```python
from build123d import *

# Parameters (mm, degrees)
SKETCH1_R           = 180
BOSS_EXTRUDE1_DEPTH = 60
FILLET1_R           = 20
SKETCH2_R           = 100
BOSS_EXTRUDE3_DEPTH = 10
SKETCH3_R           = 90
BOSS_EXTRUDE4_DEPTH = 270
SKETCH4_R           = 180
BOSS_EXTRUDE5_DEPTH = 60
FILLET2_R           = 30
BOSS_EXTRUDE6_START = 10
SKETCH6_R           = 100
BOSS_EXTRUDE6_DEPTH = 10
FILLET3_R           = 5
SKETCH9_W           = 20.845427705
SKETCH9_H           = 31.268141557
BOSS_EXTRUDE7_DEPTH = 10
SKETCH10_R          = 10
CUT_EXTRUDE2_DEPTH  = 10
CUT_EXTRUDE3_START  = 10
SKETCH12_R          = 10
CUT_EXTRUDE3_DEPTH  = 10
SKETCH13_RX         = 11.260558061
SKETCH13_RY         = 5.777483036
CUT_EXTRUDE4_DEPTH  = 30
SKETCH14_W          = 10.93815799
SKETCH14_H          = 4.07197177
SKETCH14_W_2        = 12.726253657
CUT_EXTRUDE5_DEPTH  = 30
FILLET4_START       = -31
FILLET4_DEPTH       = 62
FILLET4_START_2     = -9.089801569
FILLET4_2_DEPTH     = 40.089801569
CUT_EXTRUDE6_DEPTH  = 10
CUT_EXTRUDE7_DEPTH  = 10


with BuildPart() as part:
    # Sketch1 → Boss-Extrude1 (new body)
    with BuildSketch(Plane(origin=(0, 0, 0), x_dir=(1, 0, 0), z_dir=(0, 1, 0))):
        with Locations(Location((0, 0, 0), (0, 0, 90))):
            Circle(SKETCH1_R)
    extrude(amount=BOSS_EXTRUDE1_DEPTH)

    # Fillet1
    fillet1_edges = [part.edges().sort_by_distance(p)[0] for p in [
        (0, 0, 180),
    ]]
    fillet(fillet1_edges, radius=FILLET1_R)

    # Sketch2 → Boss-Extrude3 (add)
    with BuildSketch(Plane(origin=(0, 60, 0), x_dir=(1, 0, 0), z_dir=(0, 1, 0))):
        with Locations(Location((0, 0, 0), (0, 0, 270))):
            Circle(SKETCH2_R)
    extrude(amount=BOSS_EXTRUDE3_DEPTH)

    # Sketch3 → Boss-Extrude4 (add)
    with BuildSketch(Plane(origin=(0, 70, 0), x_dir=(1, 0, 0), z_dir=(0, 1, 0))):
        with Locations(Location((0, 0, 0), (0, 0, 270))):
            Circle(SKETCH3_R)
    extrude(amount=BOSS_EXTRUDE4_DEPTH)

    # Sketch4 → Boss-Extrude5 (add)
    with BuildSketch(Plane(origin=(0, 340, 0), x_dir=(1, 0, 0), z_dir=(0, 1, 0))):
        with Locations(Location((0, 0, 0), (0, 0, 90))):
            Circle(SKETCH4_R)
    extrude(amount=BOSS_EXTRUDE5_DEPTH)

    # Fillet2
    fillet2_edges = [part.edges().sort_by_distance(p)[0] for p in [
        (0, 400, 180),
    ]]
    fillet(fillet2_edges, radius=FILLET2_R)

    # Sketch6 → Boss-Extrude6 (add)
    with BuildSketch(Plane.XZ.offset(-340).offset(BOSS_EXTRUDE6_START)):
        with Locations(Location((0, 0, 0), (0, 0, 90))):
            Circle(SKETCH6_R)
    extrude(amount=-BOSS_EXTRUDE6_DEPTH)

    # Fillet3
    fillet3_edges = [part.edges().sort_by_distance(p)[0] for p in [
        (0, 330, -100),
        (0, 70, -100),
    ]]
    fillet(fillet3_edges, radius=FILLET3_R)

    # Sketch9 → Boss-Extrude7 (add)
    with BuildSketch(Plane(origin=(0, 60, 0), x_dir=(1, 0, 0), z_dir=(0, 1, 0))):
        with Locations((-19.512515422, -149.90314923)):
            Rectangle(SKETCH9_W, SKETCH9_H)
        with Locations((19.656209668, -149.671177345)):
            Rectangle(SKETCH9_W, SKETCH9_H)
    extrude(amount=BOSS_EXTRUDE7_DEPTH)

    # Sketch10 → Cut-Extrude2 (cut)
    with BuildSketch(Plane.XY.offset(180)):
        with Locations((0, 355)):
            Circle(SKETCH10_R)
    extrude(amount=-CUT_EXTRUDE2_DEPTH, mode=Mode.SUBTRACT)

    # Sketch12 → Cut-Extrude3 (cut)
    with BuildSketch(Plane.XY.offset(-180).offset(CUT_EXTRUDE3_START)):
        with Locations((0, 355)):
            Circle(SKETCH12_R)
    extrude(amount=-CUT_EXTRUDE3_DEPTH, mode=Mode.SUBTRACT)

    # Sketch13 → Cut-Extrude4 (cut)
    with BuildSketch(Plane.ZY.offset(29.935229274)):
        with Locations((149.903149231, 70)):
            Ellipse(SKETCH13_RX, SKETCH13_RY)
    extrude(amount=-CUT_EXTRUDE4_DEPTH, mode=Mode.SUBTRACT)

    # Sketch14 → Cut-Extrude5 (cut)
    with BuildSketch(Plane(origin=(30.07892352, 0, 0), x_dir=(0, 0, -1), z_dir=(1, 0, 0))):
        with Locations((-159.836169129, 67.964014115)):
            Rectangle(SKETCH14_W, SKETCH14_H)
        with Locations((-140.400233395, 67.964014115)):
            Rectangle(SKETCH14_W_2, SKETCH14_H)
    extrude(amount=-CUT_EXTRUDE5_DEPTH, mode=Mode.SUBTRACT)

    # Fillet4: read off the stored shape, not the designer's step
    # Fillet4 outline → Fillet4 (cut)
    with BuildSketch(Plane.YZ.offset(FILLET4_START)):
        with BuildLine():
            Line((70, 165.537220009), (68, 165.537220009))
            ThreePointArc((68, 165.537220009), (69.414213562, 164.951433572), (70, 163.537220009))
            Line((70, 163.537220009), (70, 165.537220009))
        make_face()
        with BuildLine():
            Line((70, 161.163707292), (70, 162.751420247))
            ThreePointArc((70, 162.751420247), (69.666591866, 161.645765891), (68.777528446, 160.908745692))
            add(Edge.make_bspline(
                [(68.777528446, 160.908745692), (69.381765186, 161.163707292), (70, 161.163707292)],
                knots=[6.055563227, 6.055563227, 6.055563227, 6.283185307, 6.283185307, 6.283185307], degree=2, weights=[0.927415097, 0.957557219, 1]))
        make_face()
        with BuildLine():
            Line((70, 154.367090134), (68, 154.367090134))
            ThreePointArc((68, 154.367090134), (69.414213562, 153.781303696), (70, 152.367090134))
            Line((70, 152.367090134), (70, 154.367090134))
        make_face()
        with BuildLine():
            add(Edge.make_bspline(
                [(70, 138.642591169), (69.381765186, 138.642591169), (68.777528446, 138.897552769)],
                knots=[3.141592654, 3.141592654, 3.141592654, 3.369214734, 3.369214734, 3.369214734], degree=2, weights=[1, 0.957557219, 0.927415097]))
            ThreePointArc((68.777528446, 138.897552769), (69.666591866, 138.16053257), (70, 137.054878214))
            Line((70, 137.054878214), (70, 138.642591169))
        make_face()
        with BuildLine():
            ThreePointArc((70, 148.763360224), (69.414213562, 147.349146661), (68, 146.763360224))
            Line((68, 146.763360224), (70, 146.763360224))
            Line((70, 146.763360224), (70, 148.763360224))
        make_face()
        with BuildLine():
            Line((65.92802823, 134.269078452), (64.862948862, 134.269078452))
            ThreePointArc((64.862948862, 134.269078452), (64.409662828, 134.095965635), (63.92802823, 134.037106567))
            Line((63.92802823, 134.037106567), (65.92802823, 134.037106567))
            Line((65.92802823, 134.037106567), (65.92802823, 134.269078452))
        make_face()
        with BuildLine():
            ThreePointArc((70, 136.269078452), (69.414213562, 134.85486489), (68, 134.269078452))
            Line((68, 134.269078452), (70, 134.269078452))
            Line((70, 134.269078452), (70, 136.269078452))
        make_face()
    extrude(amount=FILLET4_DEPTH, mode=Mode.SUBTRACT)

    # Fillet4 2 outline → Fillet4 2 (cut)
    with BuildSketch(Plane.YZ.offset(FILLET4_START_2)):
        with BuildLine():
            ThreePointArc((63.92802823, 165.305248124), (65.342241792, 164.719461686), (65.92802823, 163.305248124))
            Line((65.92802823, 163.305248124), (65.92802823, 165.305248124))
            Line((65.92802823, 165.305248124), (63.92802823, 165.305248124))
        make_face()
        with BuildLine():
            Line((65.92802823, 134.269078452), (65.92802823, 136.037106567))
            ThreePointArc((65.92802823, 136.037106567), (65.641189236, 135.005079741), (64.862948862, 134.269078452))
            Line((64.862948862, 134.269078452), (65.92802823, 134.269078452))
        make_face()
    extrude(amount=FILLET4_2_DEPTH, mode=Mode.SUBTRACT)

    # Sketch22 → Cut-Extrude6 (cut)
    with BuildSketch(Plane(origin=(0, 60, 0), x_dir=(1, 0, 0), z_dir=(0, 1, 0))):
        Polygon((127.423760752, -18.872499432), (107.1351894, -64.521784974), (113.629623838, -67.40820028), (133.91819519, -21.758914738), align=None)
        Polygon((137.220873331, -23.883738258), (116.932301979, -69.5330238), (123.677729052, -72.530991388), (143.966300404, -26.881705846), align=None)
        Polygon((148.265392154, -28.776757418), (127.858476847, -74.692316859), (134.98259987, -77.858593758), (155.389515177, -31.943034317), align=None)
    extrude(amount=-CUT_EXTRUDE6_DEPTH, mode=Mode.SUBTRACT)

    # Sketch24 → Cut-Extrude7 (cut)
    with BuildSketch(Plane(origin=(0, 60, 0), x_dir=(1, 0, 0), z_dir=(0, 1, 0))):
        Polygon((111.713779985, 58.505093082), (105.578926162, 52.370239259), (74.729375507, 83.219789913), (80.86422933, 89.354643737), align=None)
        Polygon((115.569973817, 62.361286914), (84.720423162, 93.210837569), (90.154150834, 98.644565241), (121.003701489, 67.795014586), align=None)
        Polygon((93.930128704, 100.831618279), (123.985216943, 70.77653004), (128.873539941, 75.664853038), (98.818451702, 105.719941277), align=None)
    extrude(amount=-CUT_EXTRUDE7_DEPTH, mode=Mode.SUBTRACT)


solid = part.part
```
Check sheet for the modelled part. Datum: model origin and axes. Units: mm. A direction names the side the tool comes from. Coordinates: 2 decimals unless noted, no trailing zeros. Order: outer loops, then holes, each group sorted by start corner. A loop starts at its lowest first (then second) coordinate and runs counter-clockwise, first axis right, second up. Notation, with made-up numbers: M 17,69.5 L 58,69.5 A29 cw 58,93.5 Z; hole C -36.5,27 d2. An arc over 180 degrees is marked long. Write each question's results on one line, items separated by ' | '. Start each with the question number.
1. Cross-section at B-B on y = 198. Record the cut outline in (x, z), and give its area (3 significant figures).
2. Cross-section at A-A on z = 0. Record the cut outline in (x, y), and give its area (3 significant figures).
3. Material ranges on probe 1 along Y at (x, z) = (10, 106.5); probe 2 along Y at (x, z) = (0, 175.25); probe 3 along Y at (x, z) = (0, 172), recorded low to high.
4. Access from +Z, -Z, +X, -X, +Y, -Y to the whole of each face (thin tool, end or side, straight path). Record for faces 4 (the face through (68.941, 39.72, -166.274)), 5 (the face through (96.07, 55.07, -74.15)), 6 (the face through (-1.302, 364.915, -174.93)), 7 (the face through (0, 355, 170)).
5. Mould release check, pull along Z, two halves, no side actions. Record for faces 1 (the face through (-9.09, 64, 150)), 2 (the face through (68.941, 354.79, -166.274)), 3 (the face through (103, 50, -81)): +Z half, -Z half, draft (parallel to the pull), parting line (faces both ways), or undercut.
6. Cross-section at C-C on y = 355. Record the cut outline in (x, z), and give its area (3 significant figures).
7. Go/stop test with flat-tipped pins: P1, Ø2.5, axis at x = -15, y = 62.5, coming from the -Z side; P2, Ø0.6, axis at x = 18, y = 67.5, coming from the -Z side; P3, Ø18, axis at x = 0, y = 355, coming from the -Z side. Record where each tip stops, or that it passes through.
Checks:
1) outline: C 0,0 d180 | area: 25,400 mm²
2) outline: M -180,20 A20 ccw -160,0 L 160,0 A20 ccw 180,20 L 180,60 L 100,60 L 100,65 A5 ccw 95,70 L 90,70 L 90,330 L 95,330 A5 ccw 100,335 L 100,340 L 180,340 L 180,370 A30 ccw 150,400 L -150,400 A30 ccw -180,370 L -180,340 L -100,340 L -100,335 A5 ccw -95,330 L -90,330 L -90,70 L -95,70 A5 ccw -100,65 L -100,60 L -180,60 Z | area: 93,400 mm²
3) probe 1: y = 0 to 60, 340 to 400 | probe 2: y = 7.06 to 60, 340 to 345, 365 to 386.2 | probe 3: y = 4 to 60, 340 to 345, 365 to 390.4
4) face 4: +Y, -Y | face 5: none | face 6: -Z | face 7: +Z
5) face 1: draft | face 2: parting line | face 3: undercut
6) outline: M -10,-179.72 L -10,-170 L 10,-170 L 10,-179.72 A180 ccw 10,179.72 L 10,170 L -10,170 L -10,179.72 A180 ccw Z | area: 101,000 mm²
7) P1: stops at z = -99.05 | P2: stops at z = -97.86 | P3: stops at z = -170
